from build123d import *

# Parameters (mm, degrees)
BOSS_EXTRUDE1_DEPTH      = 2.38125
F_5_16_24_TAPPED_HOLE1_D = 6.9088
SKETCH5_OUTSIDE_W        = 38.658
SKETCH5_OUTSIDE_H        = 40.622
SKETCH5_OUTSIDE_R        = 6.35
CUT_EXTRUDE2_DEPTH       = 5.7625
CUT_EXTRUDE2_TAPER       = 60


with BuildPart() as part:
    # Sketch1 → Boss-Extrude1 (new body, symmetric)
    with BuildSketch(Plane(origin=(0, 0, 0), x_dir=(1, 0, 0), z_dir=(0, 1, 0))):
        Polygon((-6.35, 3.666174209), (-6.35, -3.666174209), (0, -7.332348419), (6.35, -3.666174209), (6.35, 3.666174209), (0, 7.332348419), align=None)
    extrude(amount=BOSS_EXTRUDE1_DEPTH, both=True)

    # 5/16-24 Tapped Hole1 (through all)
    with Locations(Plane(origin=(0, 2.38125, 0), x_dir=(1, 0, 0), z_dir=(0, 1, 0))):
        with Locations((0, 0)):
            Hole(F_5_16_24_TAPPED_HOLE1_D / 2)

    # Sketch5 outside → Cut-Extrude2 (cut, through all)
    with BuildSketch(Plane(origin=(0, 2.38125, 0), x_dir=(1, 0, 0), z_dir=(0, 1, 0))):
        Rectangle(SKETCH5_OUTSIDE_W, SKETCH5_OUTSIDE_H)
        Circle(SKETCH5_OUTSIDE_R, mode=Mode.SUBTRACT)
    cut_extrude2 = extrude(amount=-CUT_EXTRUDE2_DEPTH, taper=CUT_EXTRUDE2_TAPER, mode=Mode.SUBTRACT)

    # Mirror1: Cut-Extrude2 across plane
    add(cut_extrude2.mirror(Plane.ZX), mode=Mode.SUBTRACT)


solid = part.part
For this review, take the finished solid that the model builds, in its own axes (mm). Round coordinates to 2 decimals unless told otherwise and drop trailing zeros. Write each loop counter-clockwise with the first axis right and the second up, starting at its lowest first coordinate (ties: lowest second). Pieces come first, ordered by that corner, then holes. Notation, with made-up numbers: (84, 37.5) -> (91, 37.5) arc R22 cw to (91, 43.5) -> close; hole circle Ø7 at (-26.75, 78.25). An arc over 180 degrees is marked (long way). Put each result on its own line as item: value.
Q1. Consider section A-A on y = 0.55. State the section outline as (x, z) points.
Determined:
outline: (-6.35, -3.67) -> (0, -7.33) -> (6.35, -3.67) -> (6.35, 3.67) -> (0, 7.33) -> (-6.35, 3.67) -> close; hole circle Ø6.91 at (0, 0)
Q2. The part is to be moulded in two halves that separate along X. For faces 1 (the conical face through (-0.016, -2.243, -6.589)), 2 (the cylindrical face through (0.45, -0.033, -3.425)), 3 (the conical face through (-5.714, 2.243, -3.28)), say which applies: released by +X, released by -X, zero draft, split by the parting line, or undercut.
Determined:
face 1: split by the parting line
face 2: undercut
face 3: released by -X
Q3. To check wall thickness, follow L1, parallel to Z at x = -1, y = 0.05 (1 decimal); L2, parallel to Z at x = -1.25, y = 1.15; L3, parallel to X at y = -0.8, z = 2. State the ranges of each line that lie inside material, in increasing order. Write a range as [from, to].
Determined:
L1: z = [-6.8, -3.3], [3.3, 6.8]
L2: z = [-6.61, -3.22], [3.22, 6.61]
L3: x = [-6.35, -2.82], [2.82, 6.35]
Q4. Clearance check with flat-ended pins moving along their axes: pin 1 Ø6 at (x, z) = (0, 0) entering from +Y; pin 2 Ø2 at (x, y) = (3, 0.5) entering from +Z. State where each tip first meets the part, or that it passes through.
Determined:
pin 1: passes through
pin 2: stops at z = 6.18
